Design review of the part built by this model. Coordinates are the model's own, in mm. A direction names the side the tool comes from. Give positions to 0.01 mm unless a question says otherwise; leave off trailing zeros. Loops run counter-clockwise (first coordinate to the right, second up) from the corner with the lowest first, then second, coordinate; pieces in that order, holes last. Notation, with made-up numbers: M 21,17.5 L 53,17.5 A27 cw 53,43.5 Z; hole C 12.5,83 d9. An arc over 180 degrees is marked long. Use CSV: the item, a comma, the result in double quotes.
from build123d import *

# Parameters (mm, degrees)
SKETCH1_W                    = 131.4
SKETCH1_H                    = 100
BASE_FLANGE1_DEPTH           = 3.175
EDGE_FLANGE1_STRIP_W         = 14.1732
EDGE_FLANGE1_STRIP_H         = 3.175
EDGE_FLANGE1_STRIP_CUT_DEPTH = 131.4
EDGE_FLANGE1_DEPTH           = 131.4
FILLET1_R                    = 2.54
SKETCH15_R                   = 12.7
MOTOR_HOLE_DEPTH             = 87.380842784
SKETCH9_R                    = 3.205
CUT_EXTRUDE1_DEPTH           = 120.102985899
SKETCH10_R                   = 3.206253706
CUT_EXTRUDE2_DEPTH           = 86.501114759


# Sheet-metal steps are written as plain solids
with BuildPart() as part:
    # Sketch1 → Base-Flange1 (new body)
    with BuildSketch(Plane(origin=(0, 0, 0), x_dir=(0, 1, 0), z_dir=(0, 0, 1))):
        Rectangle(SKETCH1_W, SKETCH1_H)
    extrude(amount=BASE_FLANGE1_DEPTH)

    # Edge-Flange1 strip (across the edge) → Edge-Flange1 strip cut (cut)
    with BuildSketch(Plane(origin=(-50, -65.7, 0), x_dir=(1, 0, 0), z_dir=(0, 1, 0))):
        with Locations((-3.175, -1.5875)):
            Rectangle(EDGE_FLANGE1_STRIP_W, EDGE_FLANGE1_STRIP_H)
    extrude(amount=EDGE_FLANGE1_STRIP_CUT_DEPTH, mode=Mode.SUBTRACT)

    # Edge-Flange1 section (across the edge) → Edge-Flange1 (add)
    with BuildSketch(Plane(origin=(-50, -65.7, 0), x_dir=(1, 0, 0), z_dir=(0, 1, 0))):
        with BuildLine():
            Line((0, 0.7366), (0, 22.225))
            Line((0, 22.225), (3.175, 22.225))
            Line((3.175, 22.225), (3.175, 0.7366))
            ThreePointArc((3.175, 0.7366), (3.390745145, 0.215745145), (3.9116, 0))
            Line((3.9116, 0), (3.9116, -3.175))
            ThreePointArc((3.9116, -3.175), (1.145681115, -2.029318885), (0, 0.7366))
        make_face()
    extrude(amount=EDGE_FLANGE1_DEPTH)

    # Fillet1
    fillet1_edges = [part.edges().sort_by_distance(p)[0] for p in [
        (-48.4125, -65.7, -22.225),
        (-48.4125, 65.7, -22.225),
        (50, 65.7, 1.5875),
        (50, -65.7, 1.5875),
    ]]
    fillet(fillet1_edges, radius=FILLET1_R)

    # Sketch15 → Motor Hole (cut, through all)
    with BuildSketch(Plane.XY.offset(3.175)):
        with Locations((-7.9, 7.8)):
            Circle(SKETCH15_R)
    extrude(amount=-MOTOR_HOLE_DEPTH, mode=Mode.SUBTRACT)

    # Sketch9 → Cut-Extrude1 (cut, through all)
    with BuildSketch(Plane.YZ.offset(-46.825)):
        with Locations(Location((53, -9.525, 0), (0, 0, 270))):
            Circle(SKETCH9_R)
    cut_extrude1 = extrude(amount=-CUT_EXTRUDE1_DEPTH, mode=Mode.SUBTRACT)

    # Mirror1: Cut-Extrude1 across plane
    add(cut_extrude1.mirror(Plane.ZX), mode=Mode.SUBTRACT)

    # Sketch10 → Cut-Extrude2 (cut, through all)
    with BuildSketch(Plane(origin=(0, 0, 0), x_dir=(1, 0, 0), z_dir=(0, 0, -1))):
        with Locations(Location((-33.3884, 53, 0), (0, 0, 180))):
            Circle(SKETCH10_R)
        with Locations(Location((37.3, 53, 0), (0, 0, 180))):
            Circle(SKETCH10_R)
    extrude(amount=-CUT_EXTRUDE2_DEPTH, mode=Mode.SUBTRACT)


solid = part.part
(1) Machinability: for faces 1 (the cylindrical face through (-48.39, -64.936, -21.501)), 2 (the flat face through (-46.825, -1, -12)), which of the approach directions +Z, -Z, +X, -X, +Y, -Y give a long, thin tool a straight path to every point of the face, cutting with its end or side? Answer none if there is none.
A:
face 1,"-Z, +X, -X, -Y"
face 2,"-Z, +X, +Y, -Y"
(2) Wall thickness on line 1 along Y through (x, z) = (37.3, 1.4); line 2 along X through (y, z) = (-30, -9.5) (3 decimals); line 3 along Z through (x, y) = (40.5, 53) (3 decimals): over which ranges is each line inside the solid? List them lowest first. Write a range as [from, to].
A:
line 1,"[-65.7, -56.21], [-49.79, 65.7]"
line 2,"[-50, -46.825]"
line 3,"[0, 3.175]"
(3) We need section B-B on y = 7.8. State the section outline as (x, z) points (3 decimals).
A:
outline,"M -50,-22.225 L -46.825,-22.225 L -46.825,-0.737 A0.737 cw -46.088,0 L -20.6,0 L -20.6,3.175 L -46.088,3.175 A3.912 ccw -50,-0.737 Z; M 4.8,0 L 50,0 L 50,3.175 L 4.8,3.175 Z"
(4) The part is to be moulded in two halves that separate along X. For faces 3 (the flat face through (12, -1, 3.175)), 4 (the cylindrical face through (49.236, 64.976, 1.61)), 5 (the cylindrical face through (-17.26, 16.383, 1.61)), say which applies: released by +X, released by -X, zero draft, split by the parting line, or undercut.
A:
face 3,"zero draft"
face 4,"released by +X"
face 5,"undercut"
(5) Clearance check with flat-ended pins moving along their axes: P1, Ø10.5, axis at y = 53, z = -9.525, coming from the +X side (3 decimals); P2, Ø7.5, axis at x = 37.3, y = -53, coming from the -Z side. State where each tip first meets the part, or that it passes through.
A:
P1,"x = -46.825"
P2,"z = 0"
(6) We need section D-D on x = -7.9. State the section outline as (y, z) points (3 decimals), then the cut area to 3 significant figures.
A:
outline,"M -65.7,0 L -4.9,0 L -4.9,3.175 L -65.7,3.175 Z; M 20.5,0 L 65.7,0 L 65.7,3.175 L 20.5,3.175 Z"
area,"337 mm²"
(7) We need section A-A on x = 37.3. State the section outline as (y, z) points (3 decimals).
A:
outline,"M -65.7,0 L -56.206,0 L -56.206,3.175 L -65.7,3.175 Z; M -49.794,0 L 65.7,0 L 65.7,3.175 L -49.794,3.175 Z"
(8) We need section C-C on y = -53. State the section outline as (x, z) points (3 decimals).
A:
outline,"M -50,-22.225 L -46.825,-22.225 L -46.825,-12.73 L -50,-12.73 Z; M -50,-6.32 L -46.825,-6.32 L -46.825,-0.737 A0.737 cw -46.088,0 L -36.595,0 L -36.595,3.175 L -46.088,3.175 A3.912 ccw -50,-0.737 Z; M -30.182,0 L 34.094,0 L 34.094,3.175 L -30.182,3.175 Z; M 40.506,0 L 50,0 L 50,3.175 L 40.506,3.175 Z"
